```python
from build123d import *

# Parameters (mm, degrees)
SKETCH1_R           = 4.5
SKETCH1_R_2         = 4
BOSS_EXTRUDE1_DEPTH = 10
BOSS_EXTRUDE2_START = -10
BOSS_EXTRUDE2_DEPTH = 10


with BuildPart() as part:
    # Sketch1 → Boss-Extrude1 (new body)
    with BuildSketch(Plane(origin=(0, 0, 0), x_dir=(1, 0, 0), z_dir=(0, 1, 0))):
        with Locations(Location((0, 0, 0), (0, 0, 270))):
            Circle(SKETCH1_R)
        with Locations(Location((0, 0, 0), (0, 0, 270))):
            Circle(SKETCH1_R_2, mode=Mode.SUBTRACT)
    extrude(amount=BOSS_EXTRUDE1_DEPTH)

    # Sketch2 → Boss-Extrude2 (add)
    with BuildSketch(Plane(origin=(0, 10, 0), x_dir=(1, 0, 0), z_dir=(0, 1, 0)).offset(BOSS_EXTRUDE2_START)):
        with BuildLine():
            ThreePointArc((-0.225, 3.041689498), (0, 3.05), (0.225, 3.041689498))
            Line((0.225, 3.041689498), (0.225, 3.993666861))
            ThreePointArc((0.225, 3.993666861), (0, 4), (-0.225, 3.993666861))
            Line((-0.225, 3.993666861), (-0.225, 3.041689498))
        make_face()
        with BuildLine():
            Line((3.571116956, -1.801977715), (2.746680375, -1.325989033))
            ThreePointArc((2.746680375, -1.325989033), (2.641377482, -1.525), (2.521680375, -1.715700465))
            Line((2.521680375, -1.715700465), (3.346116956, -2.191689147))
            ThreePointArc((3.346116956, -2.191689147), (3.464101615, -2), (3.571116956, -1.801977715))
        make_face()
        with BuildLine():
            Line((-3.346116956, -2.191689147), (-2.521680375, -1.715700465))
            ThreePointArc((-2.521680375, -1.715700465), (-2.641377482, -1.525), (-2.746680375, -1.325989033))
            Line((-2.746680375, -1.325989033), (-3.571116956, -1.801977715))
            ThreePointArc((-3.571116956, -1.801977715), (-3.464101615, -2), (-3.346116956, -2.191689147))
        make_face()
    extrude(amount=BOSS_EXTRUDE2_DEPTH)


solid = part.part
```
The model under review builds one solid part; all positions refer to its coordinate system, in mm. A direction names the side the tool comes from. Round coordinates to 2 decimals unless told otherwise and drop trailing zeros. Loops run counter-clockwise (first coordinate to the right, second up) from the corner with the lowest first, then second, coordinate; pieces in that order, holes last.
Item 1: Take a section at D-D (z = 4.25). Write out the cut boundary in (x, y).
Determined:
outline: (-1.48, 0) - (1.48, 0) - (1.48, 10) - (-1.48, 10) - close
Item 2: Take a section at C-C (x = 0). Write out the cut boundary in (y, z).
Determined:
outline: (0, -4.5) - (10, -4.5) - (10, -3.05) - (0, -3.05) - close; (0, 4) - (10, 4) - (10, 4.5) - (0, 4.5) - close
Item 3: Clearance check with flat-ended pins moving along their axes: pin 1 Ø0.5 at (y, z) = (5, -3.5) entering from +X; pin 2 Ø2 at (x, y) = (2, 2) entering from +Z; pin 3 Ø1 at (y, z) = (6, -3.5) entering from -X. State where each tip first meets the part, or that it passes through.
Determined:
pin 1: stops at x = 3.11
pin 2: stops at z = 4.39
pin 3: stops at x = -3.35
Item 4: Take a section at A-A (z = 0). Write out the cut boundary in (x, y).
Determined:
outline: (-4.5, 0) - (-4, 0) - (-4, 10) - (-4.5, 10) - close; (4, 0) - (4.5, 0) - (4.5, 10) - (4, 10) - close
Item 5: Take a section at B-B (y = 1.5). Write out the cut boundary in (x, z) (3 decimals).
Determined:
outline: circle Ø9 at (0, 0); hole (-3.571, 1.802) arc R4 ccw to (-0.225, -3.994) - (-0.225, -3.042) arc R3.05 ccw to (0.225, -3.042) - (0.225, -3.994) arc R4 ccw to (3.571, 1.802) - (2.747, 1.326) arc R3.05 ccw to (2.522, 1.716) - (3.346, 2.192) arc R4 ccw to (-3.346, 2.192) - (-2.522, 1.716) arc R3.05 ccw to (-2.747, 1.326) - close
Item 6: For faces 1 (the face through (0, 0, -4)), 2 (the face through (3.492, 4.93, -1.952)), list the 3-axis set-ups (+Z, -Z, +X, -X, +Y, -Y) from which the entire face can be reached by the end or side of a thin tool; tool diameter is ignored.
Determined:
face 1: +Z, -Z, +X, -X, -Y
face 2: +Y, -Y
Item 7: Mouldability with a two-part tool opening along X and no side actions: class faces 3 (the face through (-0.225, 4.9, -3.5)), 4 (the face through (1.352, 4.93, 4.292)), 5 (the face through (0, 10, -4)) as released by +X, released by -X, zero draft, split by the parting line, or undercut.
Determined:
face 3: undercut
face 4: split by the parting line
face 5: zero draft
Item 8: For line 1 (Z direction, x = -2, y = 7); line 2 (X direction, y = 1.5, z = 2.5); line 3 (Z direction, x = -1.5, y = 6.25), list the stretches that pass through material, from the lowest coordinate up.
Determined:
line 1: z = -4.03 to -3.46, 3.46 to 4.03
line 2: x = -3.74 to -3.12, 3.12 to 3.74
line 3: z = -4.24 to -3.71, 3.71 to 4.24
